Here's how the part is built. I have some questions about the finished solid (model axes, mm). A direction names the side the tool comes from. Round coordinates to 2 decimals unless told otherwise and drop trailing zeros. Write each loop counter-clockwise with the first axis right and the second up, starting at its lowest first coordinate (ties: lowest second). Pieces come first, ordered by that corner, then holes. Notation, with made-up numbers: (63, 59) -> (111, 59) arc R20 cw to (111, 89) -> close; hole circle Ø9 at (25, 7.5). An arc over 180 degrees is marked (long way). Put each result on its own line as item: value. Start each with the question number.
1) I want a section at B-B, the plane z = -24.5. List the corners of the cut face in (x, y) for me.
2) We'd pull the mould along X, two halves only. Please class faces 3 (the flat face through (-2, 2, -21)), 4 (the cylindrical face through (-4.75, 1.97, -25.35)), 5 (the cylindrical face through (0.1, 2, -55.5)): released by +X, released by -X, zero draft, split by the parting line, or undercut.
3) I want a section at D-D, the plane z = -18. List the corners of the cut face in (x, y) for me.
4) Which directions (+Z, -Z, +X, -X, +Y, -Y) give clear straight access to the entire face, cutting with the end or side of a thin tool? Please do faces 1 (the flat face through (0, 2, -16.5)), 2 (the flat face through (2.4, 4, -25.4)).
5) If I drill on line 1 along Z through (x, y) = (0, 1); line 2 along X through (y, z) = (2.75, 0); line 3 along Z through (x, y) = (-1, 2.55), over which ranges is the centre line in solid material (lowest first)? Write a range as [from, to].
6) Will these pins go through, and if not, where does the flat tip stop? P1, Ø2, axis at y = 1, z = -21, coming from the +X side; P2, Ø1.5, axis at x = -4.5, z = -33, coming from the -Y side.
7) I want a section at A-A, the plane y = 2.8. List the corners of the cut face in (x, z) for me, then the cut area to 3 significant figures.
8) I want a section at C-C, the plane x = -0.75. List the corners of the cut face in (y, z) for me.
from build123d import *

# Parameters (mm, degrees)
SKETCH1_R           = 1.5
SKETCH1_W           = 4
SKETCH1_H           = 10
BOSS_EXTRUDE1_DEPTH = 4


with BuildPart() as part:
    # Sketch1 → Boss-Extrude1 (new body)
    with BuildSketch(Plane(origin=(0, 0, 0), x_dir=(1, 0, 0), z_dir=(0, 1, 0))):
        with BuildLine():
            ThreePointArc((-5.490108902, 0.329703267), (0, -5.5), (5.490108902, 0.329703267))
            ThreePointArc((5.490108902, 0.329703267), (4.75, 25), (5.490108902, 49.670296733))
            ThreePointArc((5.490108902, 49.670296733), (0, 55.5), (-5.490108902, 49.670296733))
            ThreePointArc((-5.490108902, 49.670296733), (-4.75, 25), (-5.490108902, 0.329703267))
        make_face()
        Circle(SKETCH1_R, mode=Mode.SUBTRACT)
        with Locations((0, 50)):
            Circle(SKETCH1_R, mode=Mode.SUBTRACT)
        with Locations((0, 21.5)):
            Rectangle(SKETCH1_W, SKETCH1_H, mode=Mode.SUBTRACT)
    extrude(amount=BOSS_EXTRUDE1_DEPTH)


solid = part.part
Findings:
1. outline: (-4.75, 0) -> (-2, 0) -> (-2, 4) -> (-4.75, 4) -> close; (2, 0) -> (4.75, 0) -> (4.75, 4) -> (2, 4) -> close
2. face 3: undercut
2. face 4: released by -X
2. face 5: split by the parting line
3. outline: (-4.81, 0) -> (-2, 0) -> (-2, 4) -> (-4.81, 4) -> close; (2, 0) -> (4.81, 0) -> (4.81, 4) -> (2, 4) -> close
4. face 1: +Y, -Y
4. face 2: +Z, -Z, +X, -X, +Y
5. line 1: z = [-55.5, -51.5], [-48.5, -26.5], [-16.5, -1.5], [1.5, 5.5]
5. line 2: x = [-5.5, -1.5], [1.5, 5.5]
5. line 3: z = [-55.41, -51.12], [-48.88, -26.5], [-16.5, -1.12], [1.12, 5.41]
6. P1: stops at x = 4.78
6. P2: stops at y = 0
7. outline: (-5.49, -49.67) arc R5.5 ccw (long way) to (5.49, -49.67) arc R411.54 cw to (5.49, -0.33) arc R5.5 ccw (long way) to (-5.49, -0.33) arc R411.54 cw to start; hole (-2, -26.5) -> (2, -26.5) -> (2, -16.5) -> (-2, -16.5) -> close; hole circle Ø3 at (0, -50); hole circle Ø3 at (0, 0)
7. area: 541 mm2
8. outline: (0, -55.45) -> (4, -55.45) -> (4, -51.3) -> (0, -51.3) -> close; (0, -48.7) -> (4, -48.7) -> (4, -26.5) -> (0, -26.5) -> close; (0, -16.5) -> (4, -16.5) -> (4, -1.3) -> (0, -1.3) -> close; (0, 1.3) -> (4, 1.3) -> (4, 5.45) -> (0, 5.45) -> close
